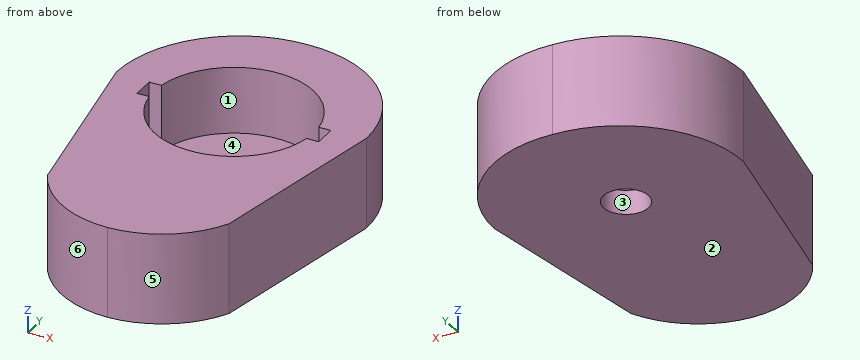
```python
from build123d import *

# Parameters (mm, degrees)
F1_DEPTH = 12.7
F2_R     = 3.175
F3_DEPTH = 9.3
F4_DEPTH = 25.4


# Not quite as in the source:
# - ends of sketch curves that miss each other by under 0.0002 mm in the source are joined


with BuildPart() as f1:
    # F0 (on Top) → F1 (new body)
    with BuildSketch(Plane.XY):
        with BuildLine():
            ThreePointArc((0, -32.75), (7.4692491087, -30.572048574), (12.7, -24.8125))
            Line((12.7, -24.8125), (17.4625, 1.9280540291))
            ThreePointArc((17.4625, 1.9280540291), (12.2942741687, 14.1229194267), (0, 19.05))
            ThreePointArc((0, 19.05), (-12.2942741687, 14.1229194267), (-17.4625, 1.9280540291))
            Line((-17.4625, 1.9280540291), (-12.7, -24.8125))
            ThreePointArc((-12.7, -24.8125), (-7.4692491087, -30.572048574), (0, -32.75))
        make_face()
    extrude(amount=F1_DEPTH)

    # F2 (on face) → F3 (cut)
    with BuildSketch(Plane.XY.offset(12.7)):
        with BuildLine():
            Line((12.7, 1.5875), (10.9985226281, 1.5875))
            ThreePointArc((10.9985226281, 1.5875), (0, 11.1125), (-10.9985226281, 1.5875))
            Line((-10.9985226281, 1.5875), (-12.7, 1.5875))
            Line((-12.7, 1.5875), (-12.7, 0))
            Line((-12.7, 0), (-12.7, -1.5875))
            Line((-12.7, -1.5875), (-10.9985226281, -1.5875))
            ThreePointArc((-10.9985226281, -1.5875), (0, -11.1125), (10.9985226281, -1.5875))
            Line((10.9985226281, -1.5875), (12.7, -1.5875))
            Line((12.7, -1.5875), (12.7, 0))
            Line((12.7, 0), (12.7, 1.5875))
        make_face()
        Circle(F2_R, mode=Mode.SUBTRACT)
    extrude(amount=-F3_DEPTH, mode=Mode.SUBTRACT)

    # F4 (cut): a face of the model
    f4_faces = [f1.faces().sort_by_distance(p)[0] for p in [
        (0, 0, 12.7),
    ]]
    extrude(f4_faces, amount=-F4_DEPTH, mode=Mode.SUBTRACT)


solid = f1.part
```
Here's how the part is built. I have some questions about the finished solid (model axes, mm). Face numbers are marked on the shaded views. A direction names the side the tool comes from. Coordinates: 2 decimals unless noted, no trailing zeros. Loops run counter-clockwise (first coordinate to the right, second up) from the corner with the lowest first, then second, coordinate; pieces in that order, holes last. Notation, with made-up numbers: (18.25, 1) -> (55.25, 1) arc R24 ccw to (55.25, 23) -> close; hole circle Ø2 at (55.5, -2.75). An arc over 180 degrees is marked (long way). Return JSON: item names as keys, results as strings.
1) If we section it at B-B, the plane y = 0: Write out the boundary of the cut face in (x, z) (3 decimals), then the cut area to 3 significant figures.
Results below:
{"outline": "(-17.119, 0) -> (-3.175, 0) -> (-3.175, 3.4) -> (-12.7, 3.4) -> (-12.7, 12.7) -> (-17.119, 12.7) -> close; (3.175, 0) -> (17.119, 0) -> (17.119, 12.7) -> (12.7, 12.7) -> (12.7, 3.4) -> (3.175, 3.4) -> close", "area": "177 mm²"}
2) If we section it at D-D, the plane y = -20.5: Write out the boundary of the cut face in (x, z), then the cut area to 3 significant figures.
Results below:
{"outline": "(-13.47, 0) -> (13.47, 0) -> (13.47, 12.7) -> (-13.47, 12.7) -> close", "area": "342 mm²"}
3) For the marked faces 1 and 2, which set-ups out of +Z, -Z, +X, -X, +Y, -Y let a thin tool reach every point of the face, with its end or its side?
Results below:
{"face 1": "+Z", "face 2": "-Z, +X, -X, +Y, -Y"}
4) Thinking about a two-plate mould opening in X: for the marked faces 3, 4, 5 and 6, which applies, +X half, -X half, draft (parallel to the pull), parting line (faces both ways), or undercut?
Results below:
{"face 3": "undercut", "face 4": "undercut", "face 5": "+X half", "face 6": "-X half"}
5) Will these pins go through, and if not, where does the flat tip stop? pin 1 (6 mm diameter, centred on y = 13.5, z = 7, fed in from -X); pin 2 (5 mm diameter, centred on x = 0, y = 0, fed in from -Z); pin 3 (1.5 mm diameter, centred on x = -2, z = 2.5, fed in from +Y); pin 4 (5 mm diameter, centred on y = 13.5, z = 5, fed in from -X).
Results below:
{"pin 1": "x = -15.12", "pin 2": "through", "pin 3": "y = 19.02", "pin 4": "x = -14.81"}
6) If we section it at C-C, the plane x = -8: Write out the boundary of the cut face in (y, z).
Results below:
{"outline": "(-30.22, 0) -> (17.2, 0) -> (17.2, 12.7) -> (7.71, 12.7) -> (7.71, 3.4) -> (-7.71, 3.4) -> (-7.71, 12.7) -> (-30.22, 12.7) -> close"}
7) I need wall thicknesses on line 1 (Y direction, x = 0, z = 2.15) (3 decimals); line 2 (Z direction, x = 0.5, y = 3.5); line 3 (X direction, y = -3, z = 8). Which ranges of each line are inside material? Lowest first, please. Write a range as from..to.
Results below:
{"line 1": "-32.75..-3.175, 3.175..19.05", "line 2": "0..3.4", "line 3": "-16.58..-10.7, 10.7..16.58"}
